from build123d import *

# Parameters (mm, degrees)
SKETCH1_R             = 11
SKETCH1_W             = 5.65685425
SKETCH1_H             = 5.65685425
BOSS_EXTRUDE1_DEPTH   = 5
F_2_0MM_DOWEL_HOLE1_D = 2
SKETCH4_R             = 1.7
CUT_EXTRUDE1_DEPTH    = 2.5
CIRPATTERN1_COUNT     = 4


with BuildPart() as part:
    # Sketch1 → Boss-Extrude1 (new body)
    with BuildSketch(Plane(origin=(0, 0, 0), x_dir=(0, 1, 0), z_dir=(0, 0, 1))):
        with Locations(Location((0, 0, 0), (0, 0, 270))):
            Circle(SKETCH1_R)
        Rectangle(SKETCH1_W, SKETCH1_H, mode=Mode.SUBTRACT)
    extrude(amount=BOSS_EXTRUDE1_DEPTH)

    # Ø2.0mm Dowel Hole1 (through all)
    with Locations(Plane.XY.offset(5)):
        with Locations((8, 0), (0, 8), (-8, 0), (0, -8)):
            Hole(F_2_0MM_DOWEL_HOLE1_D / 2)

    # Sketch4 → Cut-Extrude1 (cut)
    with BuildSketch(Plane.XY.offset(5)):
        with Locations((-8, 0)):
            Circle(SKETCH4_R)
    cut_extrude1 = extrude(amount=-CUT_EXTRUDE1_DEPTH, mode=Mode.SUBTRACT)

    # CirPattern1: Cut-Extrude1 ×4 about axis
    cirpattern1_axis = Axis((0, 0, 0), (0, 0, 1))
    for i in range(1, CIRPATTERN1_COUNT):
        add(cut_extrude1.rotate(cirpattern1_axis, i * 360 / CIRPATTERN1_COUNT), mode=Mode.SUBTRACT)


solid = part.part
CAD build for the part. Positions are in the model's coordinates, mm. A direction names the side the tool comes from. Give positions to 0.01 mm unless a question says otherwise; leave off trailing zeros. Loops run counter-clockwise (first coordinate to the right, second up) from the corner with the lowest first, then second, coordinate; pieces in that order, holes last. Notation, with made-up numbers: M -23.75,-18.5 L 28.25,-18.5 A22 ccw 28.25,16.5 Z; hole C 43.25,6.5 d7. An arc over 180 degrees is marked long. Answer in a Markdown table with one row per item. Add a question column.
Item 1: Band-saw the part on A-A on x = 0. Give the cut face in (y, z), then the cut area to 3 significant figures.
Item 2: Band-saw the part on C-C on z = 3.45. Give the cut face in (x, y), then the cut area to 3 significant figures.
Item 3: Probe probe 1 along Y at (x, z) = (1.5, 3.7); probe 2 along Y at (x, z) = (7, 3.2). List the from-to ranges inside material, lowest first.
Item 4: Mould opens along Y. For faces 4 (the face through (2.828, 0, 2)), 5 (the face through (0, 2.828, 2)), 6 (the face through (0, -5, 5)), 7 (the face through (-2.38, -10.74, 2.46)) say: +Y half, -Y half, draft (parallel to the pull), parting line (faces both ways), or undercut.
Item 5: Drop flat-ended pins along their axis: P1, Ø3, axis at x = 0, y = -8, coming from the +Z side; P2, Ø1, axis at x = -6.5, z = 0.5, coming from the +Y side. Give the stop position or say it passes through.
Item 6: Band-saw the part on D-D on y = 7.5. Give the cut face in (x, z), then the cut area to 3 significant figures.
Item 7: Tool access for faces 1 (the face through (0, -2.828, 2)), 2 (the face through (7, 1, 2.5)), 3 (the face through (0, -5, 0)): list every direction of +Z, -Z, +X, -X, +Y, -Y with a clear straight run to the whole face (end or side of a thin tool).
Reply:
| question | item | result |
|---|---|---|
| 1 | outline | M -11,0 L -9,0 L -9,2.5 L -9.7,2.5 L -9.7,5 L -11,5 Z; M -7,0 L -2.83,0 L -2.83,5 L -6.3,5 L -6.3,2.5 L -7,2.5 Z; M 2.83,0 L 7,0 L 7,2.5 L 6.3,2.5 L 6.3,5 L 2.83,5 Z; M 9,0 L 11,0 L 11,5 L 9.7,5 L 9.7,2.5 L 9,2.5 Z |
| 1 | area | 54.7 mm^2 |
| 2 | outline | C 0,0 d22; hole C -8,0 d3.4; hole M -2.83,-2.83 L 2.83,-2.83 L 2.83,2.83 L -2.83,2.83 Z; hole C 0,-8 d3.4; hole C 0,8 d3.4; hole C 8,0 d3.4 |
| 2 | area | 312 mm^2 |
| 3 | probe 1 | y = -10.9 to -8.8, -7.2 to -2.83, 2.83 to 7.2, 8.8 to 10.9 |
| 3 | probe 2 | y = -8.49 to -1.37, 1.37 to 8.49 |
| 4 | face 4 | undercut |
| 4 | face 5 | undercut |
| 4 | face 6 | draft |
| 4 | face 7 | parting line |
| 5 | P1 | stops at z = 2.5 |
| 5 | P2 | stops at y = 9.22 |
| 6 | outline | M -8.05,0 L -0.87,0 L -0.87,2.5 L -1.62,2.5 L -1.62,5 L -8.05,5 Z; M 0.87,0 L 8.05,0 L 8.05,5 L 1.62,5 L 1.62,2.5 L 0.87,2.5 Z |
| 6 | area | 68.0 mm^2 |
| 7 | face 1 | +Z, -Z |
| 7 | face 2 | +Z |
| 7 | face 3 | -Z, +X, -X, +Y, -Y |
